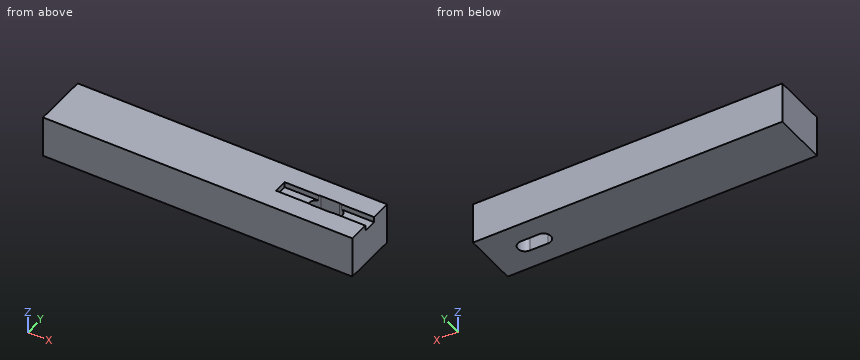
```python
from build123d import *

# Parameters (mm, degrees)
SKETCH1_W           = 24.634
SKETCH1_H           = 13
BOSS_EXTRUDE1_DEPTH = 10
SKETCH4_W           = 82.5
SKETCH4_H           = 13
BOSS_EXTRUDE4_DEPTH = 15
SKETCH5_W           = 28
SKETCH5_H           = 3.5
BOSS_EXTRUDE5_DEPTH = 15
CUT_EXTRUDE1_DEPTH  = 26
SKETCH7_W           = 32.5
SKETCH7_H           = 5
CUT_EXTRUDE2_DEPTH  = 2
SKETCH8_W           = 10
SKETCH8_H           = 13
CUT_EXTRUDE3_DEPTH  = 25.634
SKETCH9_W           = 15
SKETCH9_H           = 3.5
BOSS_EXTRUDE6_DEPTH = 54.5
SKETCH10_W          = 15
SKETCH10_H          = 20
BOSS_EXTRUDE7_DEPTH = 30


with BuildPart() as part:
    # Sketch1 → Boss-Extrude1 (new body)
    with BuildSketch(Plane.XY):
        with Locations((12.317, 6.5)):
            Rectangle(SKETCH1_W, SKETCH1_H)
    extrude(amount=BOSS_EXTRUDE1_DEPTH)

    # Sketch4 → Boss-Extrude4 (add)
    with BuildSketch(Plane.XY.offset(10)):
        with Locations((41.25, 6.5)):
            Rectangle(SKETCH4_W, SKETCH4_H)
    extrude(amount=BOSS_EXTRUDE4_DEPTH)

    # Sketch5 → Boss-Extrude5 (add)
    with BuildSketch(Plane.XY.offset(25)):
        with Locations((68.5, -1.75)):
            Rectangle(SKETCH5_W, SKETCH5_H)
        with Locations((68.5, 14.75)):
            Rectangle(SKETCH5_W, SKETCH5_H)
    extrude(amount=-BOSS_EXTRUDE5_DEPTH)

    # Sketch6 → Cut-Extrude1 (cut, through all)
    with BuildSketch(Plane.XY.offset(25)):
        with BuildLine():
            Line((63.16, 9.16), (69.84, 9.16))
            ThreePointArc((69.84, 9.16), (72.5, 6.5), (69.84, 3.84))
            Line((69.84, 3.84), (63.16, 3.84))
            ThreePointArc((63.16, 3.84), (60.5, 6.5), (63.16, 9.16))
        make_face()
    extrude(amount=-CUT_EXTRUDE1_DEPTH, mode=Mode.SUBTRACT)

    # Sketch7 → Cut-Extrude2 (cut)
    with BuildSketch(Plane.XY.offset(25)):
        with Locations((66.25, 6.5)):
            Rectangle(SKETCH7_W, SKETCH7_H)
    extrude(amount=-CUT_EXTRUDE2_DEPTH, mode=Mode.SUBTRACT)

    # Sketch8 → Cut-Extrude3 (cut, through all)
    with BuildSketch(Plane(origin=(24.634, 0, 0), x_dir=(0, 0, -1), z_dir=(1, 0, 0))):
        with Locations((-5, 6.5)):
            Rectangle(SKETCH8_W, SKETCH8_H)
    extrude(amount=-CUT_EXTRUDE3_DEPTH, mode=Mode.SUBTRACT)

    # Sketch9 → Boss-Extrude6 (add)
    with BuildSketch(Plane.ZY.offset(-54.5)):
        with Locations((17.5, 14.75)):
            Rectangle(SKETCH9_W, SKETCH9_H)
        with Locations((17.5, -1.75)):
            Rectangle(SKETCH9_W, SKETCH9_H)
    extrude(amount=BOSS_EXTRUDE6_DEPTH)

    # Sketch10 → Boss-Extrude7 (add)
    with BuildSketch(Plane.ZY):
        with Locations((17.5, 6.5)):
            Rectangle(SKETCH10_W, SKETCH10_H)
    extrude(amount=BOSS_EXTRUDE7_DEPTH)


solid = part.part
```
Here's how the part is built. I have some questions about the finished solid (model axes, mm). Round coordinates to 2 decimals unless told otherwise and drop trailing zeros. Order: outer loops, then holes, each group sorted by start corner. A loop starts at its lowest first (then second) coordinate and runs counter-clockwise, first axis right, second up. Notation, with made-up numbers: M -19.75,86 L 10.25,86 A23 ccw 10.25,107 Z; hole C 8.5,48.25 d7. An arc over 180 degrees is marked long. One line per question, with ' | ' between items.
1) For pin 1 Ø2.5 at (x, y) = (77, 5.5) entering from +Z; pin 2 Ø0.6 at (y, z) = (7, 24) entering from +X, each with a flat end and sliding along its axis, tell me the tip position at first contact or that it passes through.
Working result:
pin 1: z = 23 | pin 2: x = 50
2) I want a section at A-A, the plane x = 66. Write out the boundary of the cut face in (y, z).
Working result:
outline: M -3.5,10 L 3.84,10 L 3.84,25 L -3.5,25 Z; M 9.16,10 L 16.5,10 L 16.5,25 L 9.16,25 Z
3) I want a section at B-B, the plane z = 13.75. Write out the boundary of the cut face in (x, y).
Working result:
outline: M -30,-3.5 L 82.5,-3.5 L 82.5,16.5 L -30,16.5 Z; hole M 63.16,3.84 L 69.84,3.84 A2.66 ccw 69.84,9.16 L 63.16,9.16 A2.66 ccw Z
4) I want a section at C-C, the plane y = 6.5. Write out the boundary of the cut face in (x, z).
Working result:
outline: M -30,10 L 60.5,10 L 60.5,23 L 50,23 L 50,25 L -30,25 Z; M 72.5,10 L 82.5,10 L 82.5,23 L 72.5,23 Z
5) I need wall thicknesses on line 1 along Y through (x, z) = (65, 16.5); line 2 along X through (y, z) = (6.5, 10.5); line 3 along Z through (x, y) = (73.5, 4.75). Which ranges of each line are inside material? Lowest first, please.
Working result:
line 1: -3.5 to 3.84, 9.16 to 16.5 | line 2: -30 to 60.5, 72.5 to 82.5 | line 3: 10 to 23
